from build123d import *

# Parameters (mm, degrees)
BOSS_EXTRUDE1_DEPTH     = 82.55
CUT_EXTRUDE1_DEPTH      = 110.433918417
CUT_EXTRUDE1_DEPTH_BACK = 110.433918417


with BuildPart() as part:
    # Sketch1 → Boss-Extrude1 (new body)
    with BuildSketch(Plane(origin=(0, 0, 0), x_dir=(1, 0, 0), z_dir=(0, 1, 0))):
        with BuildLine():
            Line((0, 0), (0, -50.8))
            Line((0, -50.8), (12.7, -50.8))
            ThreePointArc((12.7, -50.8), (23.859231637, -23.859231637), (50.8, -12.7))
            Line((50.8, -12.7), (50.8, 0))
            Line((50.8, 0), (0, 0))
        make_face()
    extrude(amount=BOSS_EXTRUDE1_DEPTH)

    # Sketch2 → Cut-Extrude1 (cut, two sides: drawn at the far end of the back side and taken through both)
    with BuildSketch(Plane.XY.offset(-CUT_EXTRUDE1_DEPTH_BACK)):
        Polygon((-144.148728282, 226.698728282), (0, 82.55), (50.8, 31.75), (194.948728282, -112.398728282), (483.246184846, 175.898728282), (144.148728282, 514.996184846), align=None)
    extrude(amount=CUT_EXTRUDE1_DEPTH + CUT_EXTRUDE1_DEPTH_BACK, mode=Mode.SUBTRACT)


solid = part.part
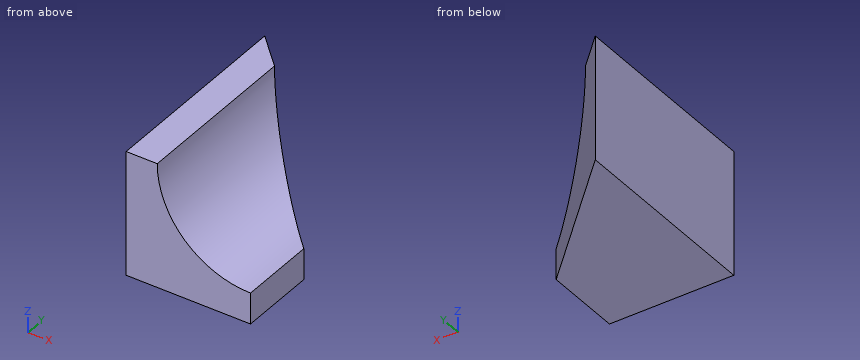
Work out the finished part from the listing and answer in its coordinate system (mm). Give positions to 0.01 mm unless a question says otherwise; leave off trailing zeros. Loops run counter-clockwise (first coordinate to the right, second up) from the corner with the lowest first, then second, coordinate; pieces in that order, holes last. Notation, with made-up numbers: (28, -21) -> (85, -21) arc R19 cw to (85, -7) -> close; hole circle Ø8 at (-8, 46). An arc over 180 degrees is marked (long way). Use a Markdown table: item, result. Add a question column.
1) The part is cut by section C-C, the plane z = 10.5. Determine the outline of the cut face in (x, y), plus the area to 3 significant figures.
2) The part is cut by section B-B, the plane x = 5.5. Determine the outline of the cut face in (y, z), plus the area to 3 significant figures.
3) The part is cut by section A-A, the plane y = 13. Determine the outline of the cut face in (x, z), plus the area to 3 significant figures.
4) Consider line 1 along Y through (x, z) = (29, 6); line 2 along Y through (x, z) = (25, 20.5); line 3 along X through (y, z) = (11, 47). Determine where each line is inside the solid, lowest interval first.
5) Each of these flat-tipped pins is pushed along its axis until it touches: P1, Ø8, axis at x = 23, z = 29, coming from the +Y side; P2, Ø1, axis at y = 70.5, z = 23, coming from the +X side; P3, Ø6, axis at x = 40.5, y = 15, coming from the +Z side. Where does it stop, or does it pass through?
Reported:
| question | item | result |
|---|---|---|
| 1 | outline | (0, 0) -> (50.8, 0) -> (50.8, 31.75) -> (0, 82.55) -> close |
| 1 | area | 2,900 mm^2 |
| 2 | outline | (0, 0) -> (77.05, 0) -> (77.05, 50.8) -> (0, 50.8) -> close |
| 2 | area | 3,910 mm^2 |
| 3 | outline | (0, 0) -> (50.8, 0) -> (50.8, 12.7) arc R38.1 cw to (12.7, 50.8) -> (0, 50.8) -> close |
| 3 | area | 1,440 mm^2 |
| 4 | line 1 | y = 0 to 53.55 |
| 4 | line 2 | y = 0 to 57.55 |
| 4 | line 3 | x = 0 to 12.89 |
| 5 | P1 | stops at y = 63.55 |
| 5 | P2 | stops at x = 12.55 |
| 5 | P3 | stops at z = 15.1 |
